from build123d import *

# Parameters (mm, degrees)
SKETCH_1_R      = 2.5
SKETCH_1_R_2    = 2
EXTRUDE_1_DEPTH = 137
EXTRUDE_2_DEPTH = 10


with BuildPart() as part:
    # 草圖1 → 填料-伸長1 (new, symmetric)
    with BuildSketch(Plane(origin=(0, 0, 0), x_dir=(0, 0, -1), z_dir=(1, 0, 0))):
        Circle(SKETCH_1_R)
        Circle(SKETCH_1_R_2, mode=Mode.SUBTRACT)
    extrude(amount=EXTRUDE_1_DEPTH, both=True)

    # 草圖3 → 填料-伸長2 (add)
    with BuildSketch(Plane(origin=(120, 0, 0), x_dir=(0, 0, -1), z_dir=(1, 0, 0))):
        with BuildLine():
            Line((2.5, 0), (2.5, -10))
            Line((2.5, -10), (0.5, -14.289013841))
            Line((0.5, -14.289013841), (0.5, -53))
            ThreePointArc((0.5, -53), (-1, -54.5), (-2.5, -53))
            Line((-2.5, -53), (-2.5, -40))
            Line((-2.5, -40), (-12.5, -40))
            Line((-12.5, -40), (-12.5, -36))
            Line((-12.5, -36), (-7.5, -36))
            ThreePointArc((-7.5, -36), (-3.964466094, -34.535533906), (-2.5, -31))
            Line((-2.5, -31), (-2.5, 0))
            ThreePointArc((-2.5, 0), (0, -2.5), (2.5, 0))
        make_face()
    extrude_2 = extrude(amount=-EXTRUDE_2_DEPTH)

    # 鏡射1: 填料-伸長2 across plane
    add(extrude_2.mirror(Plane(origin=(0, 0, 0), x_dir=(0, 0, 1), z_dir=(1, 0, 0))))


solid = part.part
Build history of the part. All positions in model axes, mm. A direction names the side the tool comes from. Round coordinates to 2 decimals unless told otherwise and drop trailing zeros. Write each loop counter-clockwise with the first axis right and the second up, starting at its lowest first coordinate (ties: lowest second). Pieces come first, ordered by that corner, then holes. Notation, with made-up numbers: (42.25, 58.25) -> (90.25, 58.25) arc R26 cw to (90.25, 92.25) -> close; hole circle Ø8 at (-16.75, 66.25). An arc over 180 degrees is marked (long way). Use one line per item in the form item = value.
Q1. Band-saw the part on B-B, the plane x = 49.5. Write the cut outline in (y, z), then the cut area to 3 significant figures.
Conclusion:
outline = circle Ø5 at (0, 0); hole circle Ø4 at (0, 0)
area = 7.07 mm²
Q2. Drop flat-ended pins along their axis: P1, Ø3, axis at x = -114, z = 9.5, coming from the -Y side; P2, Ø6, axis at x = 16.5, z = -1, coming from the -Y side; P3, Ø5.5, axis at x = -116, z = 9.5, coming from the +Y side; P4, Ø3, axis at y = 0, z = 0, coming from the -X side. Give the stop position or say it passes through.
Conclusion:
P1 = -40
P2 = -2.5
P3 = -35.94
P4 = through
Q3. Band-saw the part on A-A, the plane y = -45. Write the cut outline in (x, z), then the cut area to 3 significant figures.
Conclusion:
outline = (-120, -0.5) -> (-110, -0.5) -> (-110, 2.5) -> (-120, 2.5) -> close; (110, -0.5) -> (120, -0.5) -> (120, 2.5) -> (110, 2.5) -> close
area = 60.0 mm²
Q4. Tool access for faces 1 (the flat face through (115, -16, 2.5)), 2 (the flat face through (-115, -5, -2.5)), 3 (the flat face through (-115, -40, 7)), 4 (the flat face through (-115, -33, -0.5)), 5 (the flat face through (137, 2, 1)): list every direction of +Z, -Z, +X, -X, +Y, -Y with a clear straight run to the whole face (end or side of a thin tool).
Conclusion:
face_1 = +Z, +X, -X, +Y
face_2 = -Z, +X, -X, +Y, -Y
face_3 = +Z, +X, -X, -Y
face_4 = -Z, +X, -X, -Y
face_5 = +Z, -Z, +X, +Y, -Y
Q5. Two-plate mould, pull along X, no slides. Class faces 6 (the cylindrical face through (1.92, 2.48, 0.33)), 7 (the flat face through (-120, -27, 2)), 8 (the flat face through (-110, -27, 2)), 9 (the flat face through (115, -47, 2.5)): released by +X, released by -X, zero draft, split by the parting line, or undercut.
Conclusion:
face_6 = undercut
face_7 = released by -X
face_8 = undercut
face_9 = zero draft
Q6. Drill centre lines: L1, parallel to Y at x = -47, z = 0; L2, parallel to X at y = -34, z = 0.25; L3, parallel to Z at x = 116, y = -29. Where is each one in solid material? Low to high.
Conclusion:
L1 = -2.5 to -2, 2 to 2.5
L2 = -120 to -110, 110 to 120
L3 = -0.5 to 2.5
